```python
from build123d import *

# Parameters (mm, degrees)
SKETCH1_R           = 125
BOSS_EXTRUDE1_DEPTH = 150
SKETCH2_R           = 121
CUT_EXTRUDE1_DEPTH  = 140
SKETCH3_R           = 1.5
SKETCH3_R_2         = 4.5
CUT_EXTRUDE2_DEPTH  = 232.840462387


with BuildPart() as part:
    # Sketch1 → Boss-Extrude1 (new body)
    with BuildSketch(Plane(origin=(0, 0, 0), x_dir=(1, 0, 0), z_dir=(0, 1, 0))):
        with Locations(Location((0, 0, 0), (0, 0, 270))):
            Circle(SKETCH1_R)
    extrude(amount=BOSS_EXTRUDE1_DEPTH)

    # Sketch2 → Cut-Extrude1 (cut)
    with BuildSketch(Plane.XZ):
        with Locations(Location((0, 0, 0), (0, 0, 270))):
            Circle(SKETCH2_R)
    extrude(amount=-CUT_EXTRUDE1_DEPTH, mode=Mode.SUBTRACT)

    # Sketch3 → Cut-Extrude2 (cut, through all)
    with BuildSketch(Plane(origin=(0, 150, 0), x_dir=(1, 0, 0), z_dir=(0, 1, 0))):
        with Locations(Location((-8, 0, 0), (0, 0, 270))):
            Circle(SKETCH3_R)
        with Locations(Location((0, 0, 0), (0, 0, 270))):
            Circle(SKETCH3_R_2)
        with Locations(Location((0, 8, 0), (0, 0, 270))):
            Circle(SKETCH3_R)
        with Locations(Location((8, 0, 0), (0, 0, 270))):
            Circle(SKETCH3_R)
        with Locations(Location((0, -8, 0), (0, 0, 270))):
            Circle(SKETCH3_R)
    extrude(amount=-CUT_EXTRUDE2_DEPTH, mode=Mode.SUBTRACT)


solid = part.part
```
Read the model definition and answer for the solid it produces. Units are mm, in the model's axes. Give positions to 0.01 mm unless a question says otherwise; leave off trailing zeros. Write each loop counter-clockwise with the first axis right and the second up, starting at its lowest first coordinate (ties: lowest second). Pieces come first, ordered by that corner, then holes. Notation, with made-up numbers: (59, 56.5) -> (82, 56.5) arc R23 cw to (82, 88.5) -> close; hole circle Ø3 at (23.25, 51). An arc over 180 degrees is marked (long way). Answer in a Markdown table with one row per item.
1) Section C-C on y = 33 is taken. Give the vertices of the cut face in (x, z), plus the area to 3 significant figures.
Results list:
| item | result |
|---|---|
| outline | circle Ø250 at (0, 0); hole circle Ø242 at (0, 0) |
| area | 3,090 mm^2 |
2) Section B-B on z = -98 is taken. Give the vertices of the cut face in (x, y).
Results list:
| item | result |
|---|---|
| outline | (-77.6, 0) -> (-70.97, 0) -> (-70.97, 140) -> (70.97, 140) -> (70.97, 0) -> (77.6, 0) -> (77.6, 150) -> (-77.6, 150) -> close |
3) Determine the mould class of faces 1 (the flat face through (102.4, 0, -65.4)), 2 (the cylindrical face through (-118.123, 69.02, 26.23)), 3 (the flat face through (2, 140, -25)), 4 (the cylindrical face through (5.5, 73.95, -124.88)) for opening direction Z: released by +Z, released by -Z, zero draft, split by the parting line, or undercut.
Results list:
| item | result |
|---|---|
| face 1 | zero draft |
| face 2 | undercut |
| face 3 | undercut |
| face 4 | split by the parting line |
4) Each of these flat-tipped pins is pushed along its axis until it touches: pin 1 Ø4 at (x, z) = (-8, 0) entering from -Y; pin 2 Ø12 at (y, z) = (48, 10.5) entering from +X; pin 3 Ø4 at (y, z) = (57.5, 15.5) entering from +X. Where does it stop, or does it pass through?
Results list:
| item | result |
|---|---|
| pin 1 | y = 140 |
| pin 2 | x = 124.92 |
| pin 3 | x = 124.27 |
5) Section A-A on x = -110 is taken. Give the vertices of the cut face in (y, z).
Results list:
| item | result |
|---|---|
| outline | (0, -59.37) -> (150, -59.37) -> (150, 59.37) -> (0, 59.37) -> (0, 50.41) -> (140, 50.41) -> (140, -50.41) -> (0, -50.41) -> close |
6) Straight lines are drawn through the part: line 1 (X direction, y = 148, z = 0); line 2 (X direction, y = 126, z = 1.5); line 3 (Y direction, x = 30.5, z = 49). For each, find the intervals that lie inside material, in ascending order. Write a range as [from, to].
Results list:
| item | result |
|---|---|
| line 1 | [-125, -9.5], [-6.5, -4.5], [4.5, 6.5], [9.5, 125] |
| line 2 | [-124.99, -120.99], [120.99, 124.99] |
| line 3 | [140, 150] |
